```python
from build123d import *

# Parameters (mm, degrees)
SKETCH_R      = 1.6
SKETCH_R_2    = 12
PAD_DEPTH     = 3
SKETCH001_W   = 42.3
SKETCH001_H   = 3
PAD001_DEPTH  = 48
SKETCH002_R   = 2
SKETCH002_W   = 15
SKETCH002_H   = 15
SKETCH002_W_2 = 3
SKETCH002_H_2 = 51
POCKET_DEPTH  = 8


with BuildPart() as part:
    # Sketch → Pad (new body)
    with BuildSketch(Plane.XY):
        Polygon((0, 0), (42.3, 0), (42.3, 42.3), (42.3, 48.3), (0, 48.3), (0, 42.3), align=None)
        with Locations((5.65, 36.65)):
            Circle(SKETCH_R, mode=Mode.SUBTRACT)
        with Locations((36.65, 36.65)):
            Circle(SKETCH_R, mode=Mode.SUBTRACT)
        with Locations((5.65, 5.65)):
            Circle(SKETCH_R, mode=Mode.SUBTRACT)
        with Locations((36.65, 5.65)):
            Circle(SKETCH_R, mode=Mode.SUBTRACT)
        with Locations((21.15, 21.15)):
            Circle(SKETCH_R_2, mode=Mode.SUBTRACT)
    extrude(amount=PAD_DEPTH)

    # Sketch001 → Pad001 (new body)
    with BuildSketch(Plane(origin=(0, 0, 0), x_dir=(1, 0, 0), z_dir=(0, 0, -1))):
        with Locations((21.15, -46.8)):
            Rectangle(SKETCH001_W, SKETCH001_H)
    extrude(amount=PAD001_DEPTH)

    # Sketch002 → Pocket (cut)
    with BuildSketch(Plane(origin=(0, 48.3, 0), x_dir=(-1, 0, 0), z_dir=(0, 1, 0))):
        with Locations((-33.3, -7)):
            Circle(SKETCH002_R)
        with Locations((-9, -7)):
            Circle(SKETCH002_R)
        with Locations((-33.3, -38)):
            Circle(SKETCH002_R)
        with Locations((-9, -38)):
            Circle(SKETCH002_R)
        with Locations((-21.15, -40.5)):
            Rectangle(SKETCH002_W, SKETCH002_H)
        with Locations((-1.5, -22.5)):
            Rectangle(SKETCH002_W_2, SKETCH002_H_2)
        with Locations((-40.8, -22.5)):
            Rectangle(SKETCH002_W_2, SKETCH002_H_2)
    extrude(amount=-POCKET_DEPTH, mode=Mode.SUBTRACT)


solid = part.part
```
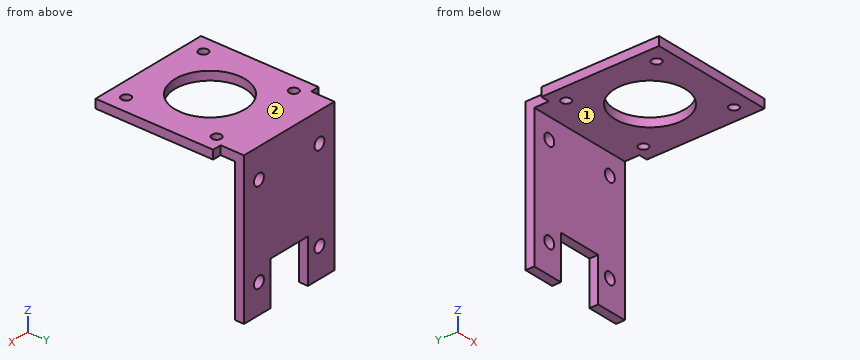
Check sheet for the modelled part. Datum: model origin and axes. Units: mm. Face numbers are marked on the shaded views. A direction names the side the tool comes from. Give positions to 0.01 mm unless a question says otherwise; leave off trailing zeros. Write each loop counter-clockwise with the first axis right and the second up, starting at its lowest first coordinate (ties: lowest second). Pieces come first, ordered by that corner, then holes. Notation, with made-up numbers: (49, 30) - (106, 30) arc R15 ccw to (106, 58) - close; hole circle Ø3 at (-24.75, 14). An arc over 180 degrees is marked (long way). Answer as a JSON object with one key per item and string values. Group by question number.
1) Access from +Z, -Z, +X, -X, +Y, -Y to the whole of each face (thin tool, end or side, straight path). Record for the marked faces 1 and 2.
2) Sectioned sample at B-B (z = -43.5). Record the cut outline in (x, y), then the cut area to 3 significant figures.
3) Sectioned sample at A-A (y = 21.15). Record the cut outline in (x, z), then the cut area to 3 significant figures.
4) Thickness scan on probe 1 along Y at (x, z) = (5.65, 1.45); probe 2 along Y at (x, z) = (21, 1); probe 3 along Y at (x, z) = (36, 2). Record the ranges inside material, lowest first. Write a range as from..to.
5) Sectioned sample at C-C (x = 26.5). Record the cut outline in (y, z), then the cut area to 3 significant figures.
6) Depth check by flat-ended pin: P1, Ø2.5, axis at x = 24.5, y = 47, coming from the -Z side; P2, Ø1.5, axis at y = 47.5, z = -42, coming from the -X side; P3, Ø6.5, axis at x = 33.3, z = -38, coming from the -Y side. Enter the tip coordinate at first touch or a pass-through.
7) Sectioned sample at D-D (y = 37.5). Record the cut outline in (x, z).
Geometry results:
{
 "1": {"face 1": "-Z, +X, -X, -Y", "face 2": "+Z, +X, -X, +Y, -Y"},
 "2": {"outline": "(3, 45.3) - (13.65, 45.3) - (13.65, 48.3) - (3, 48.3) - close; (28.65, 45.3) - (39.3, 45.3) - (39.3, 48.3) - (28.65, 48.3) - close", "area": "63.9 mm^2"},
 "3": {"outline": "(0, 0) - (9.15, 0) - (9.15, 3) - (0, 3) - close; (33.15, 0) - (42.3, 0) - (42.3, 3) - (33.15, 3) - close", "area": "54.9 mm^2"},
 "4": {"probe 1": "y = 0..4.05, 7.25..35.05, 38.25..48.3", "probe 2": "y = 0..9.15, 33.15..48.3", "probe 3": "y = 0..4.19, 7.11..35.19, 38.11..48.3"},
 "5": {"outline": "(0, 0) - (10.41, 0) - (10.41, 3) - (0, 3) - close; (31.89, 0) - (45.3, 0) - (45.3, -33) - (48.3, -33) - (48.3, 3) - (31.89, 3) - close", "area": "179 mm^2"},
 "6": {"P1": "stops at z = -33", "P2": "stops at x = 3", "P3": "stops at y = 45.3"},
 "7": {"outline": "(0, 0) - (4.29, 0) - (4.29, 3) - (0, 3) - close; (7.01, 0) - (35.29, 0) - (35.29, 3) - (7.01, 3) - close; (38.01, 0) - (42.3, 0) - (42.3, 3) - (38.01, 3) - close"}
}
